```python
from build123d import *

# Parameters (mm, degrees)
SKETCH_1_W          = 35
SKETCH_1_H          = 20
EXTRUDE_1_DEPTH     = 3.5
SKETCH_2_W          = 3.5
SKETCH_2_H          = 20
EXTRUDE_2_DEPTH     = 8
SKETCH_3_R          = 2.255
CUT_EXTRUDE_1_DEPTH = 8


with BuildPart() as part:
    # 草图1 → 凸台-拉伸1 (new body)
    with BuildSketch(Plane.XY):
        Rectangle(SKETCH_1_W, SKETCH_1_H)
    extrude(amount=EXTRUDE_1_DEPTH)

    # 草图2 → 凸台-拉伸2 (add)
    with BuildSketch(Plane.XY.offset(3.5)):
        with Locations((15.75, 0)):
            Rectangle(SKETCH_2_W, SKETCH_2_H)
    extrude(amount=EXTRUDE_2_DEPTH)

    # 草图3 → 切除-拉伸1 (cut)
    with BuildSketch(Plane.ZY.offset(-14)):
        with Locations((8.2, 5)):
            Circle(SKETCH_3_R)
        with Locations((8.2, -5)):
            Circle(SKETCH_3_R)
    extrude(amount=-CUT_EXTRUDE_1_DEPTH, mode=Mode.SUBTRACT)


solid = part.part
```
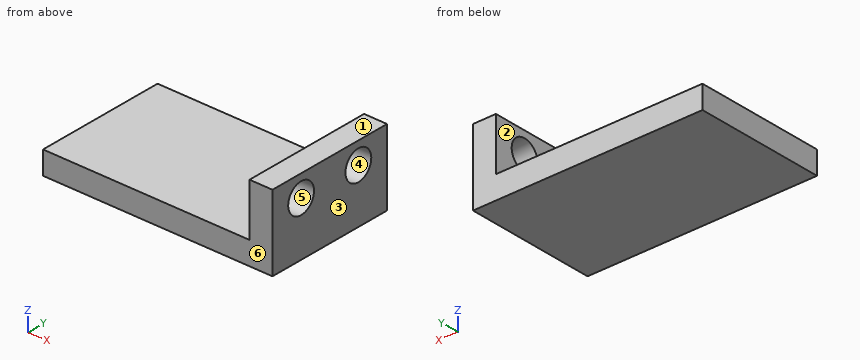
Work out the finished part from the listing and answer in its coordinate system (mm). Face numbers are marked on the shaded views. A direction names the side the tool comes from. Give positions to 0.01 mm unless a question says otherwise; leave off trailing zeros. Loops run counter-clockwise (first coordinate to the right, second up) from the corner with the lowest first, then second, coordinate; pieces in that order, holes last. Notation, with made-up numbers: (-24, 5.25) - (19, 5.25) arc R11 ccw to (19, 13.25) - close; hole circle Ø5 at (-28, 47.25). An arc over 180 degrees is marked (long way). Use CSV: the item, a comma, the result in double quotes. Start each with the question number.
(1) Each of these flat-tipped pins is pushed along its axis until it touches: pin 1 (1.5 mm diameter, centred on y = -6.5, z = 5.5, fed in from -X); pin 2 (2 mm diameter, centred on x = -5, y = 5.5, fed in from +Z). Where does it stop, or does it pass through?
(2) Find the intervals of material crossed by L1, parallel to Y at x = 14.95, z = 8.2 (3 decimals); L2, parallel to X at y = -3, z = 5.75; L3, parallel to Z at x = -14.5, y = 2.75, in increasing order.
(3) Find section C-C, the plane x = -14.5. Determine the outline of the cut face in (y, z).
(4) Find section B-B, the plane y = -5. Determine the outline of the cut face in (x, z) (3 decimals), plus the area to 3 significant figures.
(5) Find section A-A, the plane z = 8.2. Determine the outline of the cut face in (x, y) (3 decimals).
(6) Determine the mould class of the marked faces 3, 4, 5 and 6 for opening direction Y: released by +Y, released by -Y, zero draft, split by the parting line, or undercut.
(7) A tool of negligible diameter and unlimited length cuts with its end or side. For the marked faces 1 and 2, from which of +Z, -Z, +X, -X, +Y, -Y can it reach the whole face along a straight path? Write none if from no direction.
Results found:
1,pin 1,"x = 14"
1,pin 2,"z = 3.5"
2,L1,"-10 to -7.255, -2.745 to 2.745, 7.255 to 10"
2,L2,"14 to 17.5"
2,L3,"0 to 3.5"
3,outline,"(-10, 0) - (10, 0) - (10, 3.5) - (-10, 3.5) - close"
4,outline,"(-17.5, 0) - (17.5, 0) - (17.5, 5.945) - (14, 5.945) - (14, 3.5) - (-17.5, 3.5) - close; (14, 10.455) - (17.5, 10.455) - (17.5, 11.5) - (14, 11.5) - close"
4,area,"135 mm^2"
5,outline,"(14, -10) - (17.5, -10) - (17.5, -7.255) - (14, -7.255) - close; (14, -2.745) - (17.5, -2.745) - (17.5, 2.745) - (14, 2.745) - close; (14, 7.255) - (17.5, 7.255) - (17.5, 10) - (14, 10) - close"
6,face 3,"zero draft"
6,face 4,"undercut"
6,face 5,"undercut"
6,face 6,"released by -Y"
7,face 1,"+Z, +X, -X, +Y, -Y"
7,face 2,"+Z, -X, +Y, -Y"
